Can you work these out from the model? Positions are in its coordinate system, mm. Face numbers are marked on the shaded views. A direction names the side the tool comes from. Give positions to 0.01 mm unless a question says otherwise; leave off trailing zeros. Order: outer loops, then holes, each group sorted by start corner. A loop starts at its lowest first (then second) coordinate and runs counter-clockwise, first axis right, second up. Notation, with made-up numbers: M 8.5,53 L 19.5,53 A20 cw 19.5,71 Z; hole C 61.25,34 d3. An arc over 180 degrees is marked long. Answer as a JSON object with one key per item and string values.
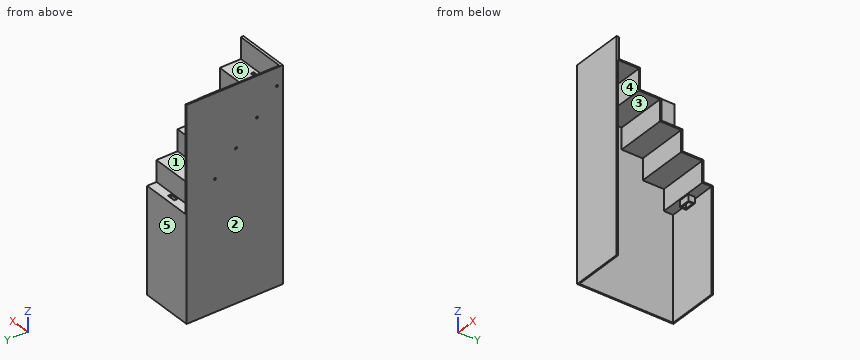
```python
from build123d import *

# Parameters (mm, degrees)
BOSS_EXTRUDE1_DEPTH = 80
SKETCH3_W           = 299
SKETCH3_H           = 299
BOSS_EXTRUDE2_DEPTH = 2
SKETCH4_W           = 82
SKETCH4_H           = 299
BOSS_EXTRUDE3_DEPTH = 2
SKETCH6_W           = 299
SKETCH6_H           = 150.5
CUT_EXTRUDE1_DEPTH  = 82
SKETCH7_W           = 132
SKETCH7_H           = 2
BOSS_EXTRUDE5_DEPTH = 80
SKETCH8_R           = 1.6
CUT_EXTRUDE2_DEPTH  = 2
CUT_EXTRUDE3_START  = -134
SKETCH9_W           = 13
SKETCH9_H           = 5
CUT_EXTRUDE3_DEPTH  = 134
SKETCH10_W          = 18
SKETCH10_H          = 10
SKETCH10_W_2        = 14
SKETCH10_H_2        = 6
BOSS_EXTRUDE6_DEPTH = 10
SKETCH11_W          = 18
SKETCH11_H          = 10
SKETCH11_W_2        = 14
SKETCH11_H_2        = 6
BOSS_EXTRUDE7_DEPTH = 10
BOSS_EXTRUDE8_DEPTH = 30


with BuildPart() as part:
    # Sketch1 → Boss-Extrude1 (new body)
    with BuildSketch(Plane(origin=(0, 0, 0), x_dir=(0, 0, -1), z_dir=(1, 0, 0))):
        Polygon((-23.931657395, -26.597399746), (-23.931657395, 6.402600254), (9.068342605, 6.402600254), (9.068342605, 39.402600254), (42.068342605, 39.402600254), (42.068342605, 72.402600254), (75.068342605, 72.402600254), (75.068342605, 105.402600254), (108.068342605, 105.402600254), (108.068342605, 138.402600254), (141.068342605, 138.402600254), (141.068342605, 171.402600254), (174.068342605, 171.402600254), (174.068342605, 204.402600254), (207.068342605, 204.402600254), (207.068342605, 237.402600254), (240.068342605, 237.402600254), (240.068342605, 272.402600254), (238.068342605, 272.402600254), (238.068342605, 239.402600254), (205.068342605, 239.402600254), (205.068342605, 206.402600254), (172.068342605, 206.402600254), (172.068342605, 173.402600254), (139.068342605, 173.402600254), (139.068342605, 140.402600254), (106.068342605, 140.402600254), (106.068342605, 107.402600254), (73.068342605, 107.402600254), (73.068342605, 74.402600254), (40.068342605, 74.402600254), (40.068342605, 41.402600254), (7.068342605, 41.402600254), (7.068342605, 8.402600254), (-25.931657395, 8.402600254), (-25.931657395, -24.597399746), (-58.931657395, -24.597399746), (-58.931657395, -26.597399746), align=None)
    extrude(amount=BOSS_EXTRUDE1_DEPTH)

    # Sketch3 → Boss-Extrude2 (add)
    with BuildSketch(Plane.ZY):
        with Locations((-90.568342605, 122.902600254)):
            Rectangle(SKETCH3_W, SKETCH3_H)
    extrude(amount=BOSS_EXTRUDE2_DEPTH)

    # Sketch4 → Boss-Extrude3 (add)
    with BuildSketch(Plane.XZ.offset(26.597399746)):
        with Locations((39, -90.568342605)):
            Rectangle(SKETCH4_W, SKETCH4_H)
    extrude(amount=BOSS_EXTRUDE3_DEPTH)

    # Sketch6 → Cut-Extrude1 (cut)
    with BuildSketch(Plane.ZY.offset(2)):
        with Locations((-90.568342605, 197.152600254)):
            Rectangle(SKETCH6_W, SKETCH6_H)
    extrude(amount=-CUT_EXTRUDE1_DEPTH, mode=Mode.SUBTRACT)

    # Sketch7 → Boss-Extrude5 (add)
    with BuildSketch(Plane(origin=(0, 0, 0), x_dir=(0, 0, -1), z_dir=(1, 0, 0))):
        with Locations((174.068342605, 120.902600254)):
            Rectangle(SKETCH7_W, SKETCH7_H)
    extrude(amount=BOSS_EXTRUDE5_DEPTH)

    # Sketch8 → Cut-Extrude2 (cut)
    with BuildSketch(Plane(origin=(0, 0, 0), x_dir=(0, 0, -1), z_dir=(1, 0, 0))):
        with Locations((-30.931657395, -19.597399746)):
            Circle(SKETCH8_R)
        with Locations((3.868342605, 11.602600254)):
            Circle(SKETCH8_R)
        with Locations((36.868342605, 44.602600254)):
            Circle(SKETCH8_R)
        with Locations((69.868342605, 77.602600254)):
            Circle(SKETCH8_R)
    extrude(amount=-CUT_EXTRUDE2_DEPTH, mode=Mode.SUBTRACT)

    # Sketch9 → Cut-Extrude3 (cut)
    with BuildSketch(Plane.XY.offset(25.931657395).offset(CUT_EXTRUDE3_START)):
        with Locations((40, -17.097399746)):
            Rectangle(SKETCH9_W, SKETCH9_H)
        with Locations((40, 112.170516798)):
            Rectangle(SKETCH9_W, SKETCH9_H)
    extrude(amount=CUT_EXTRUDE3_DEPTH, mode=Mode.SUBTRACT)

    # Sketch10 → Boss-Extrude6 (add)
    with BuildSketch(Plane.XY.offset(25.931657395)):
        with Locations((40, -17.097399746)):
            Rectangle(SKETCH10_W, SKETCH10_H)
        with Locations((40, -17.097399746)):
            Rectangle(SKETCH10_W_2, SKETCH10_H_2, mode=Mode.SUBTRACT)
    extrude(amount=-BOSS_EXTRUDE6_DEPTH)

    # Sketch11 → Boss-Extrude7 (add)
    with BuildSketch(Plane(origin=(0, 0, -108.068342605), x_dir=(-1, 0, 0), z_dir=(0, 0, -1))):
        with Locations((-40, 112.170516798)):
            Rectangle(SKETCH11_W, SKETCH11_H)
        with Locations((-40, 112.170516798)):
            Rectangle(SKETCH11_W_2, SKETCH11_H_2, mode=Mode.SUBTRACT)
    extrude(amount=BOSS_EXTRUDE7_DEPTH)

    # Sketch12 → Boss-Extrude8 (add)
    with BuildSketch(Plane(origin=(0, 0, -240.068342605), x_dir=(-1, 0, 0), z_dir=(0, 0, -1))):
        Polygon((2, -28.597399746), (2, 121.902600254), (-80, 121.902600254), (-80, 119.902600254), (0, 119.902600254), (0, -26.597399746), (-80, -26.597399746), (-80, -28.597399746), align=None)
    extrude(amount=BOSS_EXTRUDE8_DEPTH)


solid = part.part
```
1) I want a section at B-B on z = -190.5. Write out the boundary of the cut face in (x, y).
Results found:
{"outline": "M -2,-28.6 L 80,-28.6 L 80,-26.6 L 0,-26.6 L 0,119.9 L 80,119.9 L 80,121.9 L -2,121.9 Z"}
2) Thinking about a two-plate mould opening in Y: for the marked faces 4, 5 and 6, which applies, pulls with the +Y half, pulls with the -Y half, needs draft (parallel to the pull), parting line crosses it, or undercut?
Results found:
{"face 4": "undercut", "face 5": "pulls with the +Y half", "face 6": "needs draft"}
3) I want a section at D-D on x = 69. Write out the boundary of the cut face in (y, z), and give its area (3 significant figures).
Results found:
{"outline": "M -28.6,-270.07 L -26.6,-270.07 L -26.6,23.93 L 6.4,23.93 L 6.4,-9.07 L 39.4,-9.07 L 39.4,-42.07 L 72.4,-42.07 L 72.4,-75.07 L 105.4,-75.07 L 105.4,-108.07 L 119.9,-108.07 L 119.9,-270.07 L 121.9,-270.07 L 121.9,-106.07 L 107.4,-106.07 L 107.4,-73.07 L 74.4,-73.07 L 74.4,-40.07 L 41.4,-40.07 L 41.4,-7.07 L 8.4,-7.07 L 8.4,25.93 L -24.6,25.93 L -24.6,58.93 L -28.6,58.93 Z", "area": "1,610 mm²"}
4) I need wall thicknesses on L1, parallel to Y at x = 56, z = -109; L2, parallel to Y at x = 62, z = -64; L3, parallel to Z at x = 39.5, y = 68.5. Which ranges of each line are inside material? Lowest first, please.
Results found:
{"L1": "y = -28.6 to -26.6, 119.9 to 121.9", "L2": "y = -28.6 to -26.6, 72.4 to 74.4", "L3": "z = -42.07 to -40.07"}
5) I want a section at C-C on y = 68. Write out the boundary of the cut face in (x, z), and give its area (3 significant figures).
Results found:
{"outline": "M -2,-270.07 L 0,-270.07 L 0,-42.07 L 80,-42.07 L 80,-40.07 L 0,-40.07 L 0,58.93 L -2,58.93 Z", "area": "818 mm²"}
6) For the marked faces 1, 2 and 3, which set-ups out of +Z, -Z, +X, -X, +Y, -Y let a thin tool reach every point of the face, with its end or its side?
Results found:
{"face 1": "+Z, +X, +Y", "face 2": "+Z, -Z, -X, +Y, -Y", "face 3": "-Z, +X"}
7) I'm going to push flat-ended pins straight in: pin 1 Ø16.5 at (x, y) = (40, -7.5) entering from -Z; pin 2 Ø10 at (x, y) = (41.5, 51) entering from +Z; pin 3 Ø10 at (x, z) = (11, -80.5) entering from +Y; pin 4 Ø8 at (y, z) = (69, -63) entering from +X. Where does each tip first touch, or does it pass through?
Results found:
{"pin 1": "stops at z = 15.93", "pin 2": "stops at z = -40.07", "pin 3": "stops at y = 107.4", "pin 4": "stops at x = 80"}
8) I want a section at A-A on x = 42.5. Count the separate pieces of the cut face and the enclosed holes in it, and give its area (3 significant figures).
Results found:
{"separate pieces": "3", "enclosed holes": "0", "area": "1,660 mm²"}
